Model file for the job. Use its own axes, mm. A direction names the side the tool comes from. Round coordinates to 2 decimals unless told otherwise and drop trailing zeros. Use CSV: the item, a comma, the result in double quotes.
```python
from build123d import *

# Parameters (mm, degrees)
F1_DEPTH = 25


# Not quite as in the source:
# - a feature names something its author has since deleted; it is built from what else it names


with BuildPart() as f1:
    # F0 (on Front) → F1 (new body)
    with BuildSketch(Plane.XZ):
        with BuildLine():
            Line((609, -45), (609, 150))
            Line((609, 150), (-609, 150))
            Line((-609, 150), (-609, -45))
            Line((-609, -45), (-499, -45))
            ThreePointArc((-499, -45), (-481.3223304703, -52.3223304703), (-474, -70))
            Line((-474, -70), (-474, -150))
            Line((-474, -150), (474.1005301476, -150))
            Line((474.1005301476, -150), (474.0229112381, -68.9299359934))
            ThreePointArc((474.0229112381, -68.9299359934), (481.7047925737, -51.947969641), (499, -45))
            Line((499, -45), (609, -45))
        make_face()
        Polygon((-377.1515345675, -82.4994803672), (-355.4999994674, -45), (-333.8502643907, -82.5005196112), align=None, mode=Mode.SUBTRACT)
        Polygon((-258.6515341126, -82.4994803672), (-236.9999990125, -45), (-215.3502639358, -82.5005196112), align=None, mode=Mode.SUBTRACT)
        Polygon((-140.1515340625, -82.4994803672), (-118.4999989624, -45), (-96.8502638857, -82.5005196112), align=None, mode=Mode.SUBTRACT)
        Polygon((-21.651534291, -82.4994803674), (8.087e-07, -45), (21.6497358858, -82.500519611), align=None, mode=Mode.SUBTRACT)
        Polygon((96.8493649054, -82.5), (118.5, -45), (140.1506350946, -82.5), align=None, mode=Mode.SUBTRACT)
        Polygon((215.3493649054, -82.5), (237, -45), (258.6506350946, -82.5), align=None, mode=Mode.SUBTRACT)
        Polygon((333.8493649054, -82.5), (355.5, -45), (377.1506350946, -82.5), align=None, mode=Mode.SUBTRACT)
    extrude(amount=F1_DEPTH)


solid = f1.part
```
Q1. Pin check, flat tips, straight feed: pin 1 (12.5 mm diameter, centred on x = 534, y = -7.5, fed in from -Z); pin 2 (7.5 mm diameter, centred on y = -12, z = -118, fed in from -X). Stop position of each tip, or through.
From the geometry:
pin 1,"stops at z = -45"
pin 2,"stops at x = -474"
Q2. Which spindle directions (+Z, -Z, +X, -X, +Y, -Y) get a long thin tool onto all of the face, cutting with end or side? Do faces 1 (the cylindrical face through (481.513, -12.325, -52.134)), 2 (the flat face through (-474, -12, -109)). Say none if no direction does.
From the geometry:
face 1,"-Z, +X, +Y, -Y"
face 2,"-Z, -X, +Y, -Y"
Q3. Cut at A-A (y = -20). State how many separate pieces and enclosed holes the cut face has, plus the area to 3 significant figures.
From the geometry:
separate pieces,"1"
enclosed holes,"7"
area,"332,000 mm²"
Q4. Mould opens along Z. For faces 3 (the flat face through (9, -12, 150)), 4 (the flat face through (-366.477, -12.325, -64.012)), 5 (the flat face through (553, -12, -45)), 6 (the flat face through (609, -12, 51)) say: +Z half, -Z half, draft (parallel to the pull), parting line (faces both ways), or undercut.
From the geometry:
face 3,"+Z half"
face 4,"undercut"
face 5,"-Z half"
face 6,"draft"
Q5. Probe line 1 along Z through (x, y) = (-373.5, -11); line 2 along Z through (x, y) = (-1.5, -20.75); line 3 along X through (y, z) = (-10.25, -124.5). List the from-to ranges inside material, lowest first.
From the geometry:
line 1,"z = -150 to -82.5, -76.18 to 150"
line 2,"z = -150 to -82.5, -47.6 to 150"
line 3,"x = -474 to 474.08"
